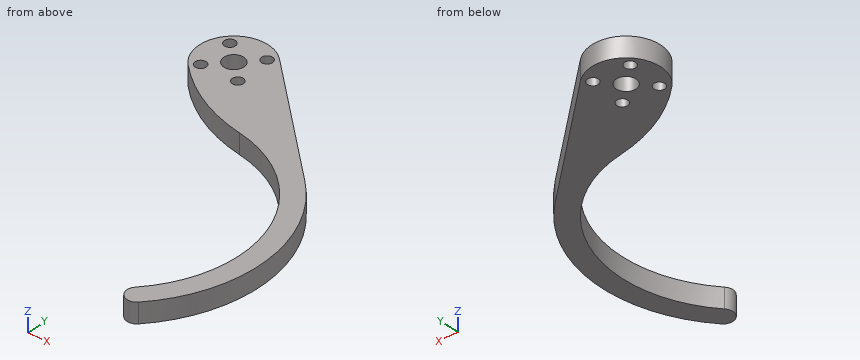
```python
from build123d import *

# Parameters (mm, degrees)
BOSS_EXTRUDE1_DEPTH = 6.35
SKETCH2_R           = 3.175
SKETCH2_R_2         = 1.75
CUT_EXTRUDE1_DEPTH  = 7.35


with BuildPart() as part:
    # Sketch1 → Boss-Extrude1 (new body)
    with BuildSketch(Plane.XY):
        with BuildLine():
            Line((-8.595455009, 68.571709933), (30.25643609, 34.276325287))
            ThreePointArc((30.25643609, 34.276325287), (45.624300947, 2.956613457), (34.427247837, -30.084597493))
            ThreePointArc((34.427247837, -30.084597493), (29.947258578, -30.386170434), (29.645685638, -25.906181175))
            ThreePointArc((29.645685638, -25.906181175), (36.792348261, 14.011424249), (4.903675305, 39.063421106))
            ThreePointArc((4.903675305, 39.063421106), (-10.270602503, 43.44261231), (-23.366607565, 52.270447493))
            ThreePointArc((-23.366607565, 52.270447493), (-24.02632087, 67.711201194), (-8.595455009, 68.571709933))
        make_face()
    extrude(amount=BOSS_EXTRUDE1_DEPTH)

    # Sketch2 → Cut-Extrude1 (cut, through all)
    with BuildSketch(Plane.XY.offset(6.35)):
        with Locations((-15.875, 60.325)):
            Circle(SKETCH2_R)
        with Locations((-10.580785461, 66.322607224)):
            Circle(SKETCH2_R_2)
        with Locations((-9.877392776, 55.030785461)):
            Circle(SKETCH2_R_2)
        with Locations((-21.169214539, 54.327392776)):
            Circle(SKETCH2_R_2)
        with Locations((-21.872607224, 65.619214539)):
            Circle(SKETCH2_R_2)
    extrude(amount=-CUT_EXTRUDE1_DEPTH, mode=Mode.SUBTRACT)


solid = part.part
```
Geometry check sheet. Reference: the model listing, model coordinates, mm. Coordinates: 2 decimals unless noted, no trailing zeros. Loops run counter-clockwise (first coordinate to the right, second up) from the corner with the lowest first, then second, coordinate; pieces in that order, holes last.
Item 1: Sectioned sample at C-C, the plane y = 59. Record the boundary of the cut face in (x, z).
Item 2: Thickness scan on line 1 (Y direction, x = -21, z = 6); line 2 (Y direction, x = -9, z = 1); line 3 (Y direction, x = 32, z = 4.5). Record the ranges inside material, lowest first.
Item 3: Sectioned sample at D-D, the plane y = 14. Record the boundary of the cut face in (x, z).
Item 4: Sectioned sample at A-A, the plane z = 3.5. Record the boundary of the cut face in (x, y) (3 decimals).
Item 5: Go/stop test with flat-tipped pins: pin 1 Ø1 at (x, z) = (32, 1.5) entering from +Y; pin 2 Ø1 at (x, z) = (4, 1.5) entering from -Y; pin 3 Ø1.5 at (y, z) = (-1.5, 2.5) entering from +X. Record where each tip stops, or that it passes through.
Item 6: Sectioned sample at B-B, the plane x = 32.5. Record the boundary of the cut face in (y, z).
Check result:
1. outline: (-26.79, 0) - (-18.76, 0) - (-18.76, 6.35) - (-26.79, 6.35) - close; (-12.99, 0) - (2.25, 0) - (2.25, 6.35) - (-12.99, 6.35) - close
2. line 1: y = 50.2 to 52.59, 56.07 to 64.1, 67.14 to 70.06
2. line 2: y = 42.87 to 53.52, 56.54 to 65.57, 67.07 to 68.91
2. line 3: y = -31.17 to -22.93, 22.93 to 32.65
3. outline: (36.8, 0) - (43.52, 0) - (43.52, 6.35) - (36.8, 6.35) - close
4. outline: (-23.367, 52.27) arc R50.8 ccw to (4.904, 39.063) arc R39.37 cw to (29.646, -25.906) arc R3.175 ccw to (34.427, -30.085) arc R45.72 ccw to (30.256, 34.276) - (-8.595, 68.572) arc R11 ccw to start; hole circle Ø3.5 at (-21.873, 65.619); hole circle Ø3.5 at (-21.169, 54.327); hole circle Ø6.35 at (-15.875, 60.325); hole circle Ø3.5 at (-10.581, 66.323); hole circle Ø3.5 at (-9.877, 55.031)
5. pin 1: stops at y = 33.14
5. pin 2: stops at y = 39.12
5. pin 3: stops at x = 45.71
6. outline: (-31.14, 0) - (-22.22, 0) - (-22.22, 6.35) - (-31.14, 6.35) - close; (22.22, 0) - (32.16, 0) - (32.16, 6.35) - (22.22, 6.35) - close
